Design review of the part built by this model. Coordinates are the model's own, in mm. A direction names the side the tool comes from. Give positions to 0.01 mm unless a question says otherwise; leave off trailing zeros. Write each loop counter-clockwise with the first axis right and the second up, starting at its lowest first coordinate (ties: lowest second). Pieces come first, ordered by that corner, then holes. Notation, with made-up numbers: (75.25, 60.25) -> (80.25, 60.25) arc R32 ccw to (80.25, 96.25) -> close; hole circle Ø10 at (46, -30.75). An arc over 180 degrees is marked (long way). Return JSON: item names as keys, results as strings. Group by question number.
from build123d import *


with BuildPart() as f1:
    # F0 (on Front) → F1 (revolve)
    with BuildSketch(Plane.XZ):
        with BuildLine():
            Line((3.5, 8.5), (3, 8.5))
            Line((3, 8.5), (3, 4.454545))
            Line((3, 4.454545), (7, 3))
            Line((7, 3), (7, 0))
            Line((7, 0), (8, 0))
            Line((8, 0), (8, 1.5))
            Line((8, 1.5), (7.5, 1.5))
            Line((7.5, 1.5), (7.5, 2.5))
            Line((7.5, 2.5), (9, 2.5))
            Line((9, 2.5), (9, 5.799573))
            ThreePointArc((9, 5.799573), (8.819067, 6.37327), (8.341743, 6.739366))
            Line((8.341743, 6.739366), (3.5, 8.5))
        make_face()
    revolve(axis=Axis((0, 0, 4.25), (0, 0, 1)))


solid = f1.part
Q1. Take a section at D-D, the plane z = 6.25. Give the boundary of the cut face in (x, y).
Q2. Tool access review of faces 1 (the face through (-7.493, 0.33, 2.007)), 2 (the face through (-4, -6, 0)), 3 (the face through (-1.73, -7.81, 0.76)): name each direction out of +Z, -Z, +X, -X, +Y, -Y from which nothing blocks a thin tool from reaching the whole face with its end or side.
Q3. Take a section at C-C, the plane z = 5. Give the boundary of the cut face in (x, y).
Q4. Mouldability with a two-part tool opening along X and no side actions: class faces 4 (the face through (-1.172, 8.923, 4.173)), 5 (the face through (3, 1, 8.5)), 6 (the face through (-3, 0, 6)), 7 (the face through (1.5, -2.884, 4.364)) as +X half, -X half, draft (parallel to the pull), parting line (faces both ways), or undercut.
Q5. Insertion check: pin 1 (3 mm diameter, centred on y = 2, z = 4.5, fed in from -X); pin 2 (1.5 mm diameter, centred on x = -2, z = 2.5, fed in from -Y); pin 3 (4 mm diameter, centred on y = 6.5, z = 4, fed in from -X). Each pin has a flat end and moves straight along its axis. Give the tip position at first contact, or say it passes through.
Q6. Take a section at A-A, the plane y = 0. Give the boundary of the cut face in (x, z), plus the area to 3 significant figures.
Q7. For L1, parallel to Y at x = 0, z = 2.15; L2, parallel to Y at x = 0, z = 1.25; L3, parallel to Z at x = 7.5, y = -1.75, list the stretches that pass through material, from the lowest coordinate up. Write a range as from..to.
Final values:
{
 "1": {"outline": "circle Ø17.79 at (0, 0); hole circle Ø6 at (0, 0)"},
 "2": {"face 1": "none", "face 2": "-Z, +X, -X, +Y, -Y", "face 3": "-Z"},
 "3": {"outline": "circle Ø18 at (0, 0); hole circle Ø6 at (0, 0)"},
 "4": {"face 4": "parting line", "face 5": "draft", "face 6": "undercut", "face 7": "undercut"},
 "5": {"pin 1": "stops at x = -8.99", "pin 2": "stops at y = -8.91", "pin 3": "stops at x = -7.79"},
 "6": {"outline": "(-9, 2.5) -> (-7.5, 2.5) -> (-7.5, 1.5) -> (-8, 1.5) -> (-8, 0) -> (-7, 0) -> (-7, 3) -> (-3, 4.45) -> (-3, 8.5) -> (-3.5, 8.5) -> (-8.34, 6.74) arc R1 ccw to (-9, 5.8) -> close; (3, 4.45) -> (7, 3) -> (7, 0) -> (8, 0) -> (8, 1.5) -> (7.5, 1.5) -> (7.5, 2.5) -> (9, 2.5) -> (9, 5.8) arc R1 ccw to (8.34, 6.74) -> (3.5, 8.5) -> (3, 8.5) -> close", "area": "55.0 mm²"},
 "7": {"L1": "y = -7.5..-7, 7..7.5", "L2": "y = -8..-7, 7..8", "L3": "z = 0..1.5, 2.5..6.97"}
}
